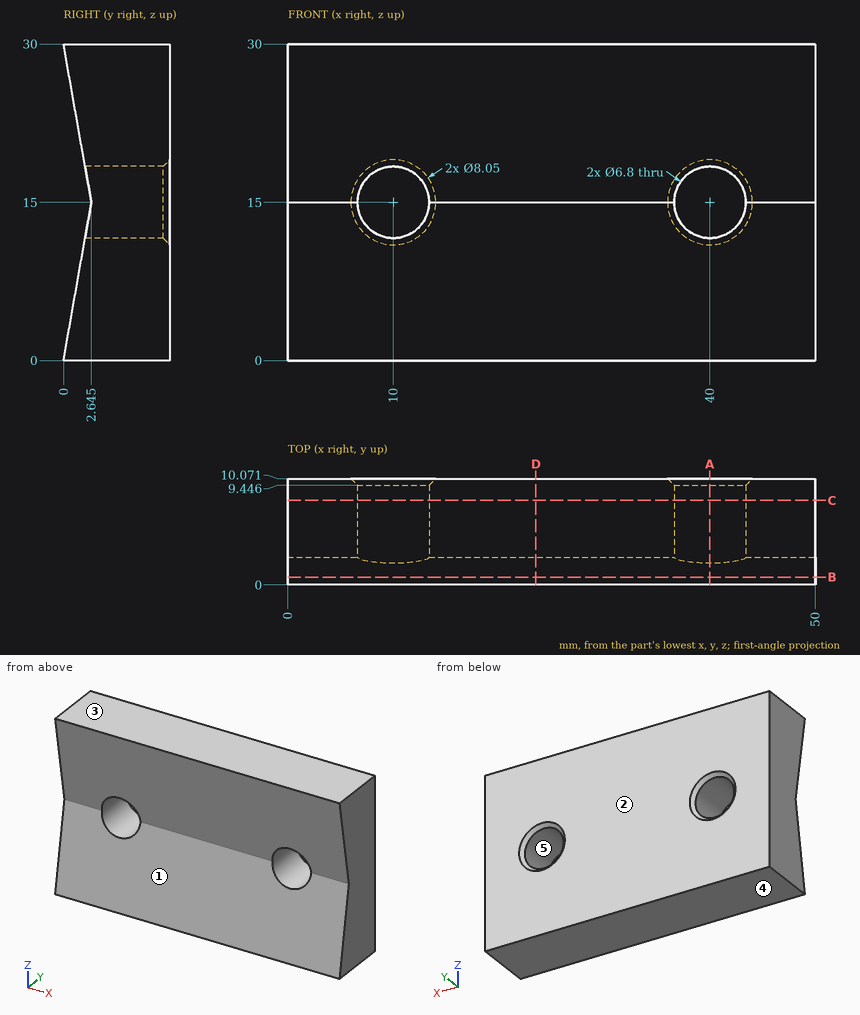
Could you check a few things on this drawing? It's one solid part, dimensions in mm from its lowest x, y, z. A direction names the side the tool comes from. Round coordinates to 2 decimals unless told otherwise and drop trailing zeros. Write each loop counter-clockwise with the first axis right and the second up, starting at its lowest first coordinate (ties: lowest second). Pieces come first, ordered by that corner, then holes. Notation, with made-up numbers: (-27.5, 70.5) -> (-11.5, 70.5) arc R27 ccw to (-11.5, 86.5) -> close; hole circle Ø8 at (61, 70.5). An arc over 180 degrees is marked (long way). Use a Markdown table: item, result.
1. If we section it at C-C (y = 8): List the corners of the cut face in (x, z) for me.
Answer key:
| item | result |
|---|---|
| outline | (0, 0) -> (50, 0) -> (50, 30) -> (0, 30) -> close; hole circle Ø6.8 at (10, 15); hole circle Ø6.8 at (40, 15) |
2. If we section it at D-D (x = 23.5): List the corners of the cut face in (y, z) for me (1 decimal).
Answer key:
| item | result |
|---|---|
| outline | (0, 0) -> (10.1, 0) -> (10.1, 30) -> (0, 30) -> (2.6, 15) -> close |
3. Please list where these lines run through material, in increasing order: probe 1 along X at (y, z) = (4.25, 14.75); probe 2 along Z at (x, y) = (40, 6.5); probe 3 along X at (y, z) = (8.25, 18).
Answer key:
| item | result |
|---|---|
| probe 1 | x = 0 to 6.61, 13.39 to 36.61, 43.39 to 50 |
| probe 2 | z = 0 to 11.6, 18.4 to 30 |
| probe 3 | x = 0 to 8.4, 11.6 to 38.4, 41.6 to 50 |
4. If we section it at B-B (y = 0.75): List the corners of the cut face in (x, z) for me.
Answer key:
| item | result |
|---|---|
| outline | (0, 0) -> (50, 0) -> (50, 4.25) -> (0, 4.25) -> close; (0, 25.75) -> (50, 25.75) -> (50, 30) -> (0, 30) -> close |
5. We'd pull the mould along Z, two halves only. Please class the marked faces 3, 4 and 5: +Z half, -Z half, draft (parallel to the pull), parting line (faces both ways), or undercut.
Answer key:
| item | result |
|---|---|
| face 3 | +Z half |
| face 4 | -Z half |
| face 5 | undercut |
6. Which directions (+Z, -Z, +X, -X, +Y, -Y) give clear straight access to the entire face, cutting with the end or side of a thin tool? Please do the marked faces 1 and 2.
Answer key:
| item | result |
|---|---|
| face 1 | +X, -X, -Y |
| face 2 | +Z, -Z, +X, -X, +Y |
7. For pin 1 Ø10 at (x, z) = (39, 15.5) entering from -Y (1 decimal); pin 2 Ø6 at (x, z) = (10, 15) entering from -Y; pin 3 Ø8 at (x, z) = (40, 15) entering from -Y, each with a flat end and sliding along its axis, tell me the tip position at first contact or that it passes through.
Answer key:
| item | result |
|---|---|
| pin 1 | stops at y = 1.7 |
| pin 2 | passes through |
| pin 3 | stops at y = 1.94 |
8. If we section it at A-A (x = 40): List the corners of the cut face in (y, z) for me (1 decimal).
Answer key:
| item | result |
|---|---|
| outline | (0, 0) -> (10.1, 0) -> (10.1, 11) -> (9.4, 11.6) -> (2, 11.6) -> close; (0, 30) -> (2, 18.4) -> (9.4, 18.4) -> (10.1, 19) -> (10.1, 30) -> close |
